Autodesk Inventor part; units mm, degrees
ref_plane "YZ Plane" through (0, 0, 0) normal (1, 0, 0) x (0, 1, 0)
ref_plane "XZ Plane" through (0, 0, 0) normal (0, 1, 0) x (-1, 0, 0)
ref_plane "XY Plane" through (0, 0, 0) normal (0, 0, 1) x (1, 0, 0)
sketch "Эскиз1" plane through (0, 0, 0) normal (0, 0, 1) x (1, 0, 0)
  line L0 (0, 0) -> (-30, 0)
  line L1 (-30, 0) -> (-30, 38)
  line L2 (-30, 38) -> (0, 38)
  line L3 (0, 38) -> (0, 0)
  dimension "d0" = 30
  dimension "d1" = 38
extrude "Выдавливание1" add sketch "Эскиз1" along normal blind 3
sketch "Эскиз2" plane through (0, 0, 0) normal (0, 0, -1) x (-1, 0, 0)
  line L0 (0, 0) -> (0, 38)
  line L1 (30, 38) -> (30, 0)
  line L2 (0, 0) -> (30, 0)
  line L3 (30, 0) -> (30, 2)
  line L4 (30, 2) -> (0, 2)
  line L5 (0, 2) -> (0, 0)
  point P0 (0, 2)
  dimension "d4" = 2
extrude "Выдавливание2" add sketch "Эскиз2" along normal blind 20
chamfer "Фаска1" distance 1 angle 45 1 edges at (-15, 2, 0)
sketch "Эскиз3" plane through (0, 0, 3) normal (0, 0, 1) x (1, 0, 0)
  circle A0 centre (-26, 34) radius 1.5
  circle A1 centre (-4, 34) radius 1.5
  circle A2 centre (-15, 14) radius 1.5
  line L0 (0, 38) -> (-30, 38)
  line L1 (-30, 38) -> (-30, 0)
  line L2 (0, 0) -> (0, 38)
  line L3 (-30, 0) -> (0, 0)
  dimension "d10" = 3
  dimension "d11" = 3
  dimension "d12" = 3
  dimension "d13" = 4
  dimension "d14" = 4
  dimension "d15" = 4
  dimension "d16" = 4
  dimension "d17" = 14
  dimension "d18" = 15
extrude "Выдавливание3" cut sketch "Эскиз3" against normal blind 20 contours A0 | A1 | A2
chamfer "Фаска2" distance 1 angle 45 3 edges at (-27.5, 34, 3) (-5.5, 34, 3) (-16.5, 14, 3)
sketch "Эскиз4" plane through (0, 0, 3) normal (0, 0, 1) x (1, 0, 0)
  line L0 (-30, 0) -> (-30, 2)
  line L1 (0, 0) -> (0, 38)
  line L2 (-30, 0) -> (0, 0)
  line L3 (0, 0) -> (0, 4)
  line L4 (0, 4) -> (-30, 4)
  line L5 (-30, 4) -> (-30, 0)
  dimension "d24" = 4
extrude "Выдавливание4" add sketch "Эскиз4" along normal blind 70
chamfer "Фаска3" distance 2 angle 45 1 edges at (-15, 4, 3)
chamfer "Фаска4" distance 1 angle 45 6 edges at (-30, 22, 3) (0, 22, 3) (-30, 0, 26.5) (-15, 0, 73) (0, 0, 26.5) (-15, 0, -20)
properties part number "camera"
Source: CAD feature listing. Evaluate the final solid. Frame: model axes, mm. A direction names the side the tool comes from. Coordinates: 2 decimals unless noted, no trailing zeros. Loops run counter-clockwise (first coordinate to the right, second up) from the corner with the lowest first, then second, coordinate; pieces in that order, holes last. Notation, with made-up numbers: (11.25, 80.5) -> (32.25, 80.5) arc R33 ccw to (32.25, 117.5) -> close; hole circle Ø1 at (79.5, -18). An arc over 180 degrees is marked (long way). One line per item, written item: value. Start each with the question number.
Q1. Section query D-D, the plane x = -11.5. Return the cut outline in (y, z), and give its area (4 significant figures).
Q2. Contact query for flat-ended pins moving along their axis: P1, Ø4, axis at x = -4, y = 34, coming from the -Z side; P2, Ø3, axis at x = -24, y = 20, coming from the +Z side; P3, Ø1.8, axis at x = -15, y = 14, coming from the +Z side; P4, Ø1, axis at x = -21.5, z = 18.5, coming from the +Y side. Output: stop coordinate, or through.
Q3. Section query C-C, the plane y = 14. Return the cut outline in (x, z).
Q4. Line query: line 1 along Y through (x, z) = (-15, 1.2); line 2 along Y through (x, z) = (-26, 0.4); line 3 along X through (y, z) = (33, 0.5). Output: solid intervals per line, ascending.
Q5. Section query A-A, the plane y = 34. Return the cut outline in (x, z), and give its area (3 significant figures).
Q6. Section query B-B, the plane x = -26. Return the cut outline in (y, z), and give its area (4 significant figures).
Q7. Set-up query: faces 1 (the face through (-15, 21, 0)), 2 (the face through (-30, 3, 30)), 3 (the face through (-15, 4, 39)). Return all of +Z, -Z, +X, -X, +Y, -Y with unobstructed straight access to the full face (end or side cutting, diameter ignored); none if empty.
Q8. Mould query, pull axis Y, two halves, no side actions, for faces 4 (the face through (-4.325, 32.536, 1.014)), 5 (the face through (0, 3, 30)), 6 (the face through (-16.5, 14.07, 1.01)), 7 (the face through (-15, 5, 4)). Classes: pulls with the +Y half, pulls with the -Y half, needs draft (parallel to the pull), parting line crosses it, or undercut.
Results:
1. outline: (0, -19) -> (1, -20) -> (2, -20) -> (2, -1) -> (3, 0) -> (38, 0) -> (38, 3) -> (6, 3) -> (4, 5) -> (4, 73) -> (1, 73) -> (0, 72) -> close
1. area: 435.5 mm^2
2. P1: z = 0
2. P2: z = 3
2. P3: through
2. P4: y = 4
3. outline: (-30, 0) -> (-16.5, 0) -> (-16.5, 2) -> (-17.5, 3) -> (-29, 3) -> (-30, 2) -> close; (-13.5, 0) -> (0, 0) -> (0, 2) -> (-1, 3) -> (-12.5, 3) -> (-13.5, 2) -> close
4. line 1: 0 to 12.5, 15.5 to 38
4. line 2: 0 to 32.5, 35.5 to 38
4. line 3: -30 to -27.12, -24.88 to -5.12, -2.88 to 0
5. outline: (-30, 0) -> (-27.5, 0) -> (-27.5, 2) -> (-28.5, 3) -> (-29, 3) -> (-30, 2) -> close; (-24.5, 0) -> (-5.5, 0) -> (-5.5, 2) -> (-6.5, 3) -> (-23.5, 3) -> (-24.5, 2) -> close; (-2.5, 0) -> (0, 0) -> (0, 2) -> (-1, 3) -> (-1.5, 3) -> (-2.5, 2) -> close
5. area: 69.0 mm^2
6. outline: (0, -19) -> (1, -20) -> (2, -20) -> (2, -1) -> (3, 0) -> (32.5, 0) -> (32.5, 2) -> (31.5, 3) -> (6, 3) -> (4, 5) -> (4, 73) -> (1, 73) -> (0, 72) -> close; (35.5, 0) -> (38, 0) -> (38, 3) -> (36.5, 3) -> (35.5, 2) -> close
6. area: 425.5 mm^2
7. face 1: -Z, +X, -X, +Y
7. face 2: +Z, -Z, -X, +Y, -Y
7. face 3: +Z, +X, -X, +Y
8. face 4: undercut
8. face 5: needs draft
8. face 6: undercut
8. face 7: pulls with the +Y half
